Source: CAD feature listing. Evaluate the final solid. Frame: model axes, mm. A direction names the side the tool comes from. Round coordinates to 2 decimals unless told otherwise and drop trailing zeros. Write each loop counter-clockwise with the first axis right and the second up, starting at its lowest first coordinate (ties: lowest second). Pieces come first, ordered by that corner, then holes. Notation, with made-up numbers: M 23.5,-24 L 65.5,-24 A21 cw 65.5,-5 Z; hole C -33,-35.5 d6. An arc over 180 degrees is marked long. Answer in a Markdown table with one row per item.
from build123d import *

# Parameters (mm, degrees)
EXTRUDE_1_DEPTH          = 12
CUT_EXTRUDE_1_DEPTH      = 12
CUT_EXTRUDE_1_DEPTH_BACK = 12


with BuildPart() as part:
    # 草图1 → 凸台-拉伸1 (new body)
    with BuildSketch(Plane.XY):
        with BuildLine():
            ThreePointArc((38.97114317, 22.5), (38.97114317, -22.5), (0, -45))
            add(Edge.make_bspline(
                [(0, -45), (-0.523588562, -45.000001824), (-1.308996546, -44.986287154), (-2.355040538, -44.936973624), (-3.138561651, -44.883613379), (-3.920631292, -44.813054932), (-4.70074178, -44.724529495), (-5.478335846, -44.617332694), (-6.252812136, -44.490834911), (-7.02353199, -44.344490532), (-7.789826844, -44.177846129), (-8.551006285, -43.990547434), (-9.306366601, -43.782344994), (-10.055199679, -43.553098452), (-10.796802122, -43.302779375), (-11.530484409, -43.031472601), (-12.255579979, -42.73937609), (-12.971454051, -42.426799279), (-13.677512056, -42.09415998), (-14.37320753, -41.741979863), (-15.05804933, -41.370878602), (-15.731608057, -40.981566772), (-16.393521567, -40.574837604), (-17.043499489, -40.151557733), (-17.681326658, -39.712657057), (-18.306865404, -39.259117879), (-18.920056659, -38.791963465), (-19.520919847, -38.312246209), (-20.109551561, -37.821035543), (-20.686123026, -37.31940579), (-21.250876386, -36.808424103), (-21.804119858, -36.289138682), (-22.346221822, -35.762567407), (-22.877603916, -35.229687052), (-23.398733251, -34.691423221), (-23.910113836, -34.148641142), (-24.412277346, -33.602137436), (-24.905773374, -33.052632959), (-25.391159289, -32.500766815), (-25.868989871, -31.947091613), (-26.339806873, -31.392070001), (-26.804128666, -30.836072544), (-27.262440122, -30.279376925), (-27.715182905, -29.7221685), (-28.162746317, -29.164542162), (-28.605458836, -28.606505484), (-29.043580492, -28.047983083), (-29.477296206, -27.488822134), (-29.90671018, -26.928798938), (-30.331841461, -26.367626442), (-30.75262073, -25.804962595), (-31.168888381, -25.240419403), (-31.580393929, -24.673572552), (-31.986796771, -24.103971433), (-32.387668279, -23.531149436), (-32.782495247, -22.954634315), (-33.170684562, -22.373958572), (-33.551569347, -21.788669334), (-34.048685337, -21.001581207), (-34.408299842, -20.403074718), (-34.641016151, -20)],
                knots=[0, 0, 0, 0, 0.03496569, 0.052447761, 0.069928514, 0.087407152, 0.104882797, 0.122354544, 0.139821494, 0.157282786, 0.174737606, 0.19218518, 0.209624761, 0.227055593, 0.244476873, 0.261887701, 0.279287021, 0.296673569, 0.314045814, 0.331401914, 0.348739666, 0.366056487, 0.383349391, 0.400614991, 0.41784952, 0.435048865, 0.452208618, 0.469324147, 0.486390681, 0.50340341, 0.520357584, 0.537248637, 0.554072295, 0.570824701, 0.587502516, 0.604103031, 0.620624249, 0.637064964, 0.653424809, 0.669704291, 0.685904798, 0.702028578, 0.718078697, 0.734058971, 0.749973875, 0.765828434, 0.781628096, 0.797378593, 0.813085806, 0.828755612, 0.844393755, 0.860005715, 0.875596595, 0.891171031, 0.906733116, 0.922286353, 0.937833634, 0.953377231, 0.968918825, 1, 1, 1, 1], degree=3))
            ThreePointArc((-34.641016151, -20), (-34.641016151, 20), (0, 40))
            add(Edge.make_bspline(
                [(0, 40), (0.4654311, 39.999999123), (1.163560176, 39.987817071), (2.093756484, 39.950846058), (2.791074225, 39.913634778), (3.488048828, 39.867790841), (4.184739053, 39.814118217), (4.881253208, 39.753364306), (5.577743667, 39.68620968), (6.274400215, 39.613258847), (6.971442786, 39.535032082), (7.669113606, 39.45195847), (8.367668884, 39.364370228), (9.067370185, 39.272498416), (9.768475628, 39.176470065), (10.471231044, 39.07630678), (11.175861244, 38.971924832), (11.882561524, 38.863136716), (12.591489567, 38.749654177), (13.302757843, 38.631092623), (14.016426662, 38.506976884), (14.732497978, 38.376748205), (15.45091006, 38.239772383), (16.171533117, 38.095348923), (16.894165968, 37.942721064), (17.618533816, 37.78108656), (18.344287177, 37.609609022), (19.071001996, 37.427429695), (19.798180969, 37.23367948), (20.525256051, 37.027491046), (21.251592153, 36.808010854), (21.976491955, 36.574410941), (22.699201797, 36.325900283), (23.41891857, 36.061735598), (24.134797494, 35.78123144), (24.845960711, 35.483769443), (25.551506534, 35.168806587), (26.250519254, 34.835882393), (26.942079336, 34.484624936), (27.625273883, 34.114755605), (28.299207181, 33.726092553), (28.963011201, 33.318552786), (29.615855866, 32.892152891), (30.256958951, 32.447008371), (30.885595446, 31.983331645), (31.50110623, 31.501428717), (32.102905932, 31.001694605), (32.690489833, 30.484607589), (33.263439702, 29.95072239), (33.821428462, 29.400662388), (34.36422361, 28.835111002), (34.891689323, 28.254802394), (35.403787201, 27.66051161), (35.900575639, 27.05304436), (36.382207825, 26.433226546), (36.848928347, 25.801893764), (37.301068575, 25.15988081), (37.739040459, 24.508011745), (38.304769224, 23.62676784), (38.709350469, 22.953441907), (38.97114317, 22.5)],
                knots=[0, 0, 0, 0, 0.031081175, 0.046622769, 0.062166366, 0.077713647, 0.093266884, 0.108828969, 0.124403405, 0.139994285, 0.155606245, 0.171244388, 0.186914194, 0.202621407, 0.218371904, 0.234171566, 0.250026125, 0.265941029, 0.281921303, 0.297971422, 0.314095202, 0.330295709, 0.346575191, 0.362935036, 0.379375751, 0.395896969, 0.412497484, 0.429175299, 0.445927705, 0.462751363, 0.479642416, 0.49659659, 0.513609319, 0.530675853, 0.547791382, 0.564951135, 0.58215048, 0.599385009, 0.616650609, 0.633943513, 0.651260334, 0.668598086, 0.685954186, 0.703326431, 0.720712979, 0.738112299, 0.755523127, 0.772944407, 0.790375239, 0.80781482, 0.825262394, 0.842717214, 0.860178506, 0.877645456, 0.895117203, 0.912592848, 0.930071486, 0.947552239, 0.96503431, 1, 1, 1, 1], degree=3))
        make_face()
    extrude(amount=EXTRUDE_1_DEPTH)

    # 草图2 → 切除-拉伸1 (cut, two sides: drawn at the far end of the back side and taken through both)
    with BuildSketch(Plane.XY.offset(-CUT_EXTRUDE_1_DEPTH_BACK)):
        with BuildLine():
            Line((9.761355821, -2.171619796), (12.585125127, -3.801923765))
            Line((12.585125127, -3.801923765), (9.585125127, -8.998076188))
            Line((9.585125127, -8.998076188), (6.761355821, -7.367772218))
            ThreePointArc((6.761355821, -7.367772218), (-8.660254038, 5), (9.761355821, -2.171619796))
        make_face()
    extrude(amount=CUT_EXTRUDE_1_DEPTH + CUT_EXTRUDE_1_DEPTH_BACK, mode=Mode.SUBTRACT)


solid = part.part
Q1. Material intervals for probe 1 along Y at (x, z) = (0, 9.5); probe 2 along X at (y, z) = (0, 2.5); probe 3 along Y at (x, z) = (-3, 4.5), sorted ascending.
Solutions:
| item | result |
|---|---|
| probe 1 | y = -45 to -10, 10 to 40 |
| probe 2 | x = -40 to -10, 10 to 45 |
| probe 3 | y = -44.89 to -9.54, 9.54 to 39.89 |
Q2. Pull-direction query (X, two-part tool) for faces 1 (the flat face through (13, -2, 12)), 2 (the cylindrical face through (39.297, -21.926, 5.916)), 3 (the cylindrical face through (-8.852, 4.652, 5.916)), 4 (the cylindrical face through (-34.93, 19.49, 5.92)); classes: pulls with the +X half, pulls with the -X half, needs draft (parallel to the pull), parting line crosses it, or undercut.
Solutions:
| item | result |
|---|---|
| face 1 | needs draft |
| face 2 | pulls with the +X half |
| face 3 | undercut |
| face 4 | pulls with the -X half |
Q3. Section A-A (y = 0). Return loops of the section in (x, z), and give its area (3 significant figures).
Solutions:
| item | result |
|---|---|
| outline | M -40,0 L -10,0 L -10,12 L -40,12 Z; M 10,0 L 45,0 L 45,12 L 10,12 Z |
| area | 780 mm2 |
Q4. Contact query for flat-ended pins moving along their axis: pin 1 Ø23 at (x, y) = (0, 0) entering from -Z; pin 2 Ø6 at (y, z) = (-24.5, 6.5) entering from -X; pin 3 Ø1.5 at (y, z) = (-27, 1.5) entering from +X; pin 4 Ø5 at (x, z) = (-6.5, 8) entering from +Y. Output: stop coordinate, or through.
Solutions:
| item | result |
|---|---|
| pin 1 | stops at z = 0 |
| pin 2 | stops at x = -33.73 |
| pin 3 | stops at x = 36.55 |
| pin 4 | stops at y = 39.8 |
Q5. Access query for faces 5 (the flat face through (11.2, -3, 5.9)), 6 (the flat face through (13, -2, 0)). Directions: +Z, -Z, +X, -X, +Y, -Y. A direction counts if a zero-diameter tool reaches every point of the face in a straight line with its end or side. Return the directions, or none.
Solutions:
| item | result |
|---|---|
| face 5 | +Z, -Z |
| face 6 | -Z, +X, -X, +Y, -Y |
